from build123d import *

# Parameters (mm, degrees)
SKETCH_1_R      = 4
EXTRUDE_1_DEPTH = 1


with BuildPart() as part:
    # 草图1 → 凸台-拉伸1 (new body)
    with BuildSketch(Plane.XY):
        with BuildLine():
            Line((-30.308871265, 18.5), (24.691128735, 18.5))
            ThreePointArc((24.691128735, 18.5), (37.414867681, 2.03528305), (34.05591144, -18.5))
            Line((34.05591144, -18.5), (-30.94408856, -18.5))
            ThreePointArc((-30.94408856, -18.5), (-38.208814547, 0.130173786), (-30.308871265, 18.5))
        make_face()
        with Locations((-17.44408856, -1.5)):
            Circle(SKETCH_1_R, mode=Mode.SUBTRACT)
        with BuildLine():
            Line((-16.94408856, -11.603927424), (-6.484848095, -11.603927424))
            Line((-6.484848095, -11.603927424), (-6.484848095, -14.383556294))
            ThreePointArc((-6.484848095, -14.383556294), (-6.906034088, -14.843943267), (-7.412736188, -15.208095416))
            Line((-7.412736188, -15.208095416), (-16.411800764, -15.208095416))
            ThreePointArc((-16.411800764, -15.208095416), (-16.710853614, -14.817070491), (-16.94408856, -14.383556294))
            Line((-16.94408856, -14.383556294), (-16.94408856, -11.603927424))
        make_face(mode=Mode.SUBTRACT)
    extrude(amount=EXTRUDE_1_DEPTH)


solid = part.part
The model under review builds one solid part; all positions refer to its coordinate system, in mm. Give positions to 0.01 mm unless a question says otherwise; leave off trailing zeros. Loops run counter-clockwise (first coordinate to the right, second up) from the corner with the lowest first, then second, coordinate; pieces in that order, holes last. Notation, with made-up numbers: (-22.75, -21) -> (11.25, -21) arc R20 cw to (11.25, 17) -> close; hole circle Ø1 at (45.5, 32). An arc over 180 degrees is marked (long way). Answer as a JSON object with one key per item and string values. Group by question number.
Q1. Wall thickness on line 1 along Y through (x, z) = (-12, 0.45); line 2 along Y through (x, z) = (-21, 0.9); line 3 along X through (y, z) = (-2.5, 0.35): over which ranges is each line inside the solid? List them lowest first.
Q2. Take a section at A-A (z = 0.3). Write out the cut boundary in (x, y).
Q3. Take a section at B-B (y = -1.5). Write out the cut boundary in (x, z), plus the area to 3 significant figures.
Q4. Take a section at C-C (x = -33). Write out the cut boundary in (y, z), plus the area to 3 significant figures.
Q5. Insertion check: pin 1 (0.5 mm diameter, centred on y = -13, z = 0.5, fed in from +X); pin 2 (6.5 mm diameter, centred on x = -17.44, y = -1.5, fed in from +Z). Each pin has a flat end and moves straight along its axis. Give the tip position at first contact, or say it passes through.
Q6. Take a section at D-D (y = -9). Write out the cut boundary in (x, z).
Q7. Draft analysis for pull direction Y (two halves, no side actions). For faces 1 (the cylindrical face through (-21.44, -1.32, 0.49)), 2 (the cylindrical face through (37.34, 2.33, 0.49)), 3 (the flat face through (1, 0, 0)), state which applies: pulls with the +Y half, pulls with the -Y half, needs draft (parallel to the pull), parting line crosses it, or undercut.
Answer below:
{
 "1": {"line 1": "y = -18.5 to -15.21, -11.6 to 18.5", "line 2": "y = -18.5 to -3.33, 0.33 to 18.5", "line 3": "x = -38.12 to -21.32, -13.57 to 38.15"},
 "2": {"outline": "(-30.94, -18.5) -> (34.06, -18.5) arc R26.1 ccw to (24.69, 18.5) -> (-30.31, 18.5) arc R26.36 ccw to start; hole circle Ø8 at (-17.44, -1.5); hole (-16.94, -14.38) arc R3.09 ccw to (-16.41, -15.21) -> (-7.41, -15.21) arc R3.02 ccw to (-6.48, -14.38) -> (-6.48, -11.6) -> (-16.94, -11.6) -> close"},
 "3": {"outline": "(-38.19, 0) -> (-21.44, 0) -> (-21.44, 1) -> (-38.19, 1) -> close; (-13.44, 0) -> (38.05, 0) -> (38.05, 1) -> (-13.44, 1) -> close", "area": "68.2 mm2"},
 "4": {"outline": "(-16.06, 0) -> (15.42, 0) -> (15.42, 1) -> (-16.06, 1) -> close", "area": "31.5 mm2"},
 "5": {"pin 1": "stops at x = 36.83", "pin 2": "passes through"},
 "6": {"outline": "(-36.74, 0) -> (37.8, 0) -> (37.8, 1) -> (-36.74, 1) -> close"},
 "7": {"face 1": "undercut", "face 2": "parting line crosses it", "face 3": "needs draft"}
}
